Input: part model. Units: mm. Frame: model coordinates. Face numbers are marked on the shaded views. A direction names the side the tool comes from. Give positions to 0.01 mm unless a question says otherwise; leave off trailing zeros. Loops run counter-clockwise (first coordinate to the right, second up) from the corner with the lowest first, then second, coordinate; pieces in that order, holes last. Notation, with made-up numbers: M 52,23 L 60,23 A20 cw 60,47 Z; hole C 30.5,78 d7. An arc over 180 degrees is marked long. One line per item, written item: value. Start each with the question number.
(1) Access query for the marked faces 1 and 2. Directions: +Z, -Z, +X, -X, +Y, -Y. A direction counts if a zero-diameter tool reaches every point of the face in a straight line with its end or side. Return the directions, or none.
(2) Ray query, line 1 along Z through (x, y) = (-9.5, -9.75); line 2 along Z through (x, y) = (-9, -14.75); line 3 along Z through (x, y) = (44, -11.5). Return the intervals inside material, ascending. Write a range as from..to.
(3) Section C-C on x = -29. Output: boundary loops of the cut face in (y, z), plus the area to 3 significant figures.
(4) Pull-direction query (Z, two-part tool) for the marked faces 3, 4 and 5; classes: released by +Z, released by -Z, zero draft, split by the parting line, or undercut.
(5) Section B-B on y = -23.5. Output: boundary loops of the cut face in (x, z), plus the area to 3 significant figures.
(6) Pin query (flat end, axial travel): P1, Ø6, axis at x = -5.5, y = -15.5, coming from the +Z side; P2, Ø12.5, axis at x = -26, y = -6.5, coming from the +Z side; P3, Ø2, axis at x = -8, y = -18.5, coming from the -Z side. Return the tip coordinate at first contact, or that it passes through.
(7) Section D-D on z = 8.5. Output: boundary loops of the cut face in (x, y), plus the area to 3 significant figures.
(8) Section A-A on x = 4.5. Output: boundary loops of the cut face in (y, z), plus the area to 3 significant figures.
```python
from build123d import *

# Parameters (mm, degrees)
F1_DEPTH = 25.4


with BuildPart() as f1:
    # F0 (on Front) → F1 (new body)
    with BuildSketch(Plane.XZ):
        with BuildLine():
            ThreePointArc((-45.9678303927, -22.7815092248), (11.6989896867, -49.9516990089), (51.3033974856, 0))
            ThreePointArc((51.3033974856, 0), (11.4099635295, 50.0185098321), (-46.2282065968, 22.2484046263))
            Line((-46.2282065968, 22.2484046263), (-4.8995565251, 22.2484046263))
            ThreePointArc((-4.8995565251, 22.2484046263), (14.2719632564, 17.7569205485), (22.7815092248, 0))
            ThreePointArc((22.7815092248, 0), (16.1089596585, -16.1089596585), (0, -22.7815092248))
            Line((0, -22.7815092248), (-45.9678303927, -22.7815092248))
        make_face()
    extrude(amount=F1_DEPTH)


solid = f1.part
```
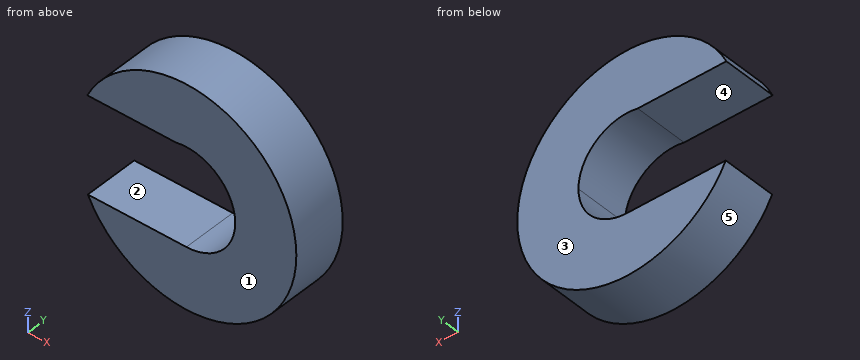
Output values:
1. face 1: +Z, -Z, +X, -X, -Y
1. face 2: -X, +Y, -Y
2. line 1: z = -50.42..-22.78, 22.25..50.42
2. line 2: z = -50.51..-22.78, 22.25..50.51
2. line 3: z = -26.38..26.38
3. outline: M -25.4,-42.32 L 0,-42.32 L 0,-22.78 L -25.4,-22.78 Z; M -25.4,22.25 L 0,22.25 L 0,42.32 L -25.4,42.32 Z
3. area: 1,010 mm²
4. face 3: zero draft
4. face 4: undercut
4. face 5: split by the parting line
5. outline: M -46.23,22.25 L -4.9,22.25 A22.78 cw long 0,-22.78 L -45.97,-22.78 A51.3 ccw long Z
5. area: 5,220 mm²
6. P1: stops at z = 51.24
6. P2: stops at z = 47.35
6. P3: stops at z = -50.82
7. outline: M 21.14,-25.4 L 50.59,-25.4 L 50.59,0 L 21.14,0 Z
7. area: 748 mm²
8. outline: M -25.4,-51.11 L 0,-51.11 L 0,-22.33 L -25.4,-22.33 Z; M -25.4,22.33 L 0,22.33 L 0,51.11 L -25.4,51.11 Z
8. area: 1,460 mm²
